Geometry: final body of the model. Coordinates: model frame, mm. Give positions to 0.01 mm unless a question says otherwise; leave off trailing zeros. Loops run counter-clockwise (first coordinate to the right, second up) from the corner with the lowest first, then second, coordinate; pieces in that order, holes last. Notation, with made-up numbers: (65, 28) -> (115, 28) arc R26 ccw to (115, 57) -> close; hole circle Ø3 at (-26.75, 71). An arc over 180 degrees is marked (long way). One line per question, with ' | ' between items. Start each with the question number.
Item 1: Section D-D on z = 3.5. Return loops of the section in (x, y), then the cut area to 3 significant figures.
Item 2: Material intervals for line 1 along Y through (x, z) = (0, 7.25); line 2 along Y through (x, z) = (-18, 6); line 3 along Y through (x, z) = (3.5, 6.5), sorted ascending. Write a range as [from, to].
Item 3: Pin query (flat end, axial travel): P1, Ø6, axis at x = 4.5, z = 5, coming from the -Y side; P2, Ø5, axis at y = 23, z = 3, coming from the -X side; P3, Ø4, axis at x = 11, z = 8.5, coming from the -Y side. Return the tip coordinate at first contact, or that it passes through.
Item 4: Section A-A on y = 8.5. Return loops of the section in (x, z).
Item 5: Section C-C on y = 0. Return loops of the section in (x, z), then the cut area to 3 significant figures.
Item 6: Section B-B on x = 11.5. Return loops of the section in (y, z).
Item 7: Mould query, pull axis X, two halves, no side actions, for faces 1 (the cylindrical face through (17.507, 0.33, 5.07)), 2 (the flat face through (16, 1, 0)), 3 (the cylindrical face through (-4.88, 37.18, 4.93)). Classes: released by +X, released by -X, zero draft, split by the parting line, or undercut.
from build123d import *

# Parameters (mm, degrees)
SKETCH_1_R     = 37.5
PAD_1_DEPTH    = 10
SKETCH_2_R     = 15
POCKET_2_DEPTH = 10.001
SKETCH_3_R     = 7.5
POCKET_3_DEPTH = 10.001
SKETCH_4_R     = 4.5
POCKET_4_DEPTH = 10.001
SKETCH_5_R     = 7.5
POCKET_5_DEPTH = 10.001
SKETCH_6_R     = 4.5
POCKET_6_DEPTH = 10.001
SKETCH_7_R     = 7.5
POCKET_7_DEPTH = 10.001
SKETCH_8_R     = 4.5
POCKET_8_DEPTH = 10.001


with BuildPart() as part:
    # Sketch_1 → Pad_1 (new body)
    with BuildSketch(Plane.XY):
        Circle(SKETCH_1_R)
    extrude(amount=PAD_1_DEPTH)

    # Sketch_2 (on Face3 of Pad_1) → Pocket_2 (cut, through all)
    with BuildSketch(Plane.XY.offset(10)):
        Circle(SKETCH_2_R)
    extrude(amount=-POCKET_2_DEPTH, mode=Mode.SUBTRACT)

    # Sketch_3 (on Face3 of Pocket_2) → Pocket_3 (cut, through all)
    with BuildSketch(Plane.XY.offset(10)):
        with Locations((25, 0)):
            Circle(SKETCH_3_R)
    extrude(amount=-POCKET_3_DEPTH, mode=Mode.SUBTRACT)

    # Sketch_4 (on Face3 of Pocket_3) → Pocket_4 (cut, through all)
    with BuildSketch(Plane.XY.offset(10)):
        with Locations((25, 0)):
            Circle(SKETCH_4_R)
    extrude(amount=-POCKET_4_DEPTH, mode=Mode.SUBTRACT)

    # Sketch_5 (on Face3 of Pocket_4) → Pocket_5 (cut, through all)
    with BuildSketch(Plane.XY.offset(10)):
        with Locations((-12.5, 21.65)):
            Circle(SKETCH_5_R)
    extrude(amount=-POCKET_5_DEPTH, mode=Mode.SUBTRACT)

    # Sketch_6 (on Face3 of Pocket_5) → Pocket_6 (cut, through all)
    with BuildSketch(Plane.XY.offset(10)):
        with Locations((-12.5, 21.65)):
            Circle(SKETCH_6_R)
    extrude(amount=-POCKET_6_DEPTH, mode=Mode.SUBTRACT)

    # Sketch_7 (on Face3 of Pocket_6) → Pocket_7 (cut, through all)
    with BuildSketch(Plane.XY.offset(10)):
        with Locations((-12.5, -21.65)):
            Circle(SKETCH_7_R)
    extrude(amount=-POCKET_7_DEPTH, mode=Mode.SUBTRACT)

    # Sketch_8 (on Face3 of Pocket_7) → Pocket_8 (cut, through all)
    with BuildSketch(Plane.XY.offset(10)):
        with Locations((-12.5, -21.65)):
            Circle(SKETCH_8_R)
    extrude(amount=-POCKET_8_DEPTH, mode=Mode.SUBTRACT)


solid = part.part
Result sheet:
1) outline: circle Ø75 at (0, 0); hole circle Ø15 at (-12.5, -21.65); hole circle Ø15 at (-12.5, 21.65); hole circle Ø30 at (0, 0); hole circle Ø15 at (25, 0) | area: 3,180 mm²
2) line 1: y = [-37.5, -15], [15, 37.5] | line 2: y = [-32.9, -26.75], [-16.55, 16.55], [26.75, 32.9] | line 3: y = [-37.34, -14.59], [14.59, 37.34]
3) P1: stops at y = -37.47 | P2: stops at x = -31.4 | P3: stops at y = -36.4
4) outline: (-36.52, 0) -> (-12.36, 0) -> (-12.36, 10) -> (-36.52, 10) -> close; (12.36, 0) -> (36.52, 0) -> (36.52, 10) -> (12.36, 10) -> close
5) outline: (-37.5, 0) -> (-15, 0) -> (-15, 10) -> (-37.5, 10) -> close; (15, 0) -> (17.5, 0) -> (17.5, 10) -> (15, 10) -> close; (32.5, 0) -> (37.5, 0) -> (37.5, 10) -> (32.5, 10) -> close | area: 300 mm²
6) outline: (-35.69, 0) -> (-9.63, 0) -> (-9.63, 10) -> (-35.69, 10) -> close; (9.63, 0) -> (35.69, 0) -> (35.69, 10) -> (9.63, 10) -> close
7) face 1: undercut | face 2: zero draft | face 3: split by the parting line
